Source: CAD feature listing. Evaluate the final solid. Frame: model axes, mm. A direction names the side the tool comes from. Round coordinates to 2 decimals unless told otherwise and drop trailing zeros. Order: outer loops, then holes, each group sorted by start corner. A loop starts at its lowest first (then second) coordinate and runs counter-clockwise, first axis right, second up. Notation, with made-up numbers: (12, 77) - (65, 77) arc R13 cw to (65, 88) - close; hole circle Ø4 at (26.25, 61). An arc over 180 degrees is marked (long way). Put each result on its own line as item: value. Start each with the question number.
1) Contact query for flat-ended pins moving along their axis: P1, Ø1.4, axis at x = 42, y = -207.5, coming from the +Z side; P2, Ø4, axis at y = -32.5, z = 39, coming from the -X side (3 decimals); P3, Ø8.5, axis at x = 48.5, z = 36.5, coming from the +Y side. Output: stop coordinate, or through.
2) Section B-B on z = 12. State how many separate pieces and enclosed holes the cut face has, then the cut area to 3 significant figures.
3) Access query for faces 1 (the face through (19, -96, 24.384)), 2 (the face through (31.75, -63, 4)), 3 (the face through (43.18, -90, 14)). Directions: +Z, -Z, +X, -X, +Y, -Y. A direction counts if a zero-diameter tool reaches every point of the face in a straight line with its end or side. Return the directions, or none.
4) Mould query, pull axis Y, two halves, no side actions, for faces 4 (the face through (20, -55.88, 17)), 5 (the face through (43.18, -203, 39)), 6 (the face through (32.258, -160, 12)), 7 (the face through (47, -177.8, 37)). Classes: +Y half, -Y half, draft (parallel to the pull), parting line (faces both ways), or undercut.
5) Line query: probe 1 along Y at (x, z) = (11, 14.5); probe 2 along X at (y, z) = (-203, 19); probe 3 along X at (y, z) = (-187, 5.5). Output: solid intervals per line, ascending. Write a range as [from, to].
6) Section C-C on z = 41. Output: boundary loops of the cut face in (x, y) (3 decimals).
7) Section D-D on x = 16. Output: boundary loops of the cut face in (y, z), then the cut area to 3 significant figures.
8) Section A-A on y = -203.2. Output: boundary loops of the cut face in (x, z).
```python
from build123d import *

# Parameters (mm, degrees)
F0_W            = 50.8
F0_H            = 44.45
F3_DEPTH        = 228.6
F4_SIZE2        = 12.7
F4_SIZE         = 25.4
F1_W            = 27.178
F1_H            = 8.89
F5_DEPTH        = 228.6
F2_W            = 4.572
F2_H            = 10.16
F6_DEPTH        = 228.6
F8_DEPTH        = 24.384
F9_W            = 2.364222
F9_H            = 0.78807
F10_DEPTH       = 12.192
F12_DEPTH       = 35.56
F14_D           = 6.35
F14_CBORE_D     = 16.51
F14_CBORE_DEPTH = 35.56


with BuildPart() as f3:
    # F0 (on Front) → F3 (new body)
    with BuildSketch(Plane.XZ):
        with Locations((25.4, 22.225)):
            Rectangle(F0_W, F0_H)
    extrude(amount=F3_DEPTH)

    # F4
    f4_edges = [f3.edges().sort_by_distance(p)[0] for p in [
        (0, -114.3, 44.45),
    ]]
    chamfer(f4_edges, length=F4_SIZE, length2=F4_SIZE2)

    # F1 (on Front) → F5 (cut)
    with BuildSketch(Plane.XZ):
        with Locations((18.161, 4.445)):
            Rectangle(F1_W, F1_H)
    extrude(amount=F5_DEPTH, mode=Mode.SUBTRACT)

    # F2 (on Front) → F6 (cut)
    with BuildSketch(Plane.XZ):
        with Locations((40.894, 39.37)):
            Rectangle(F2_W, F2_H)
    extrude(amount=F6_DEPTH, mode=Mode.SUBTRACT)

    # F7 (on face) → F8 (cut)
    with BuildSketch(Plane(origin=(0, 0, 0), x_dir=(1, 0, 0), z_dir=(0, 0, -1))):
        with BuildLine():
            ThreePointArc((32.258, 53.34), (31.514051, 55.136051), (29.718, 55.88))
            Line((29.718, 55.88), (9.398, 55.88))
            ThreePointArc((9.398, 55.88), (7.601949, 55.136051), (6.858, 53.34))
            Line((6.858, 53.34), (6.858, 7.62))
            ThreePointArc((6.858, 7.62), (7.601949, 5.823949), (9.398, 5.08))
            Line((9.398, 5.08), (29.718, 5.08))
            ThreePointArc((29.718, 5.08), (31.514051, 5.823949), (32.258, 7.62))
            Line((32.258, 7.62), (32.258, 53.34))
        make_face()
        with BuildLine():
            ThreePointArc((32.258, 118.11), (31.514051, 119.906051), (29.718, 120.65))
            Line((29.718, 120.65), (9.398, 120.65))
            ThreePointArc((9.398, 120.65), (7.601949, 119.906051), (6.858, 118.11))
            Line((6.858, 118.11), (6.858, 72.39))
            ThreePointArc((6.858, 72.39), (7.601949, 70.593949), (9.398, 69.85))
            Line((9.398, 69.85), (29.718, 69.85))
            ThreePointArc((29.718, 69.85), (31.514051, 70.593949), (32.258, 72.39))
            Line((32.258, 72.39), (32.258, 118.11))
        make_face()
        with BuildLine():
            ThreePointArc((32.258, 182.88), (31.514051, 184.676051), (29.718, 185.42))
            Line((29.718, 185.42), (9.398, 185.42))
            ThreePointArc((9.398, 185.42), (7.601949, 184.676051), (6.858, 182.88))
            Line((6.858, 182.88), (6.858, 137.16))
            ThreePointArc((6.858, 137.16), (7.601949, 135.363949), (9.398, 134.62))
            Line((9.398, 134.62), (29.718, 134.62))
            ThreePointArc((29.718, 134.62), (31.514051, 135.363949), (32.258, 137.16))
            Line((32.258, 137.16), (32.258, 182.88))
        make_face()
    extrude(amount=-F8_DEPTH, mode=Mode.SUBTRACT)

    # F9 (on face) → F10 (cut)
    with BuildSketch(Plane.YZ.offset(50.8)):
        with BuildLine():
            Line((0, 22.098), (0, 44.45))
            Line((0, 44.45), (-177.8, 44.45))
            Line((-177.8, 44.45), (-177.8, 28.448))
            ThreePointArc((-177.8, 28.448), (-175.940128, 23.957872), (-171.45, 22.098))
            Line((-171.45, 22.098), (0, 22.098))
        make_face()
        with Locations((10.441655, 33.889506)):
            Rectangle(F9_W, F9_H)
    extrude(amount=-F10_DEPTH, mode=Mode.SUBTRACT)

    # F11 (on face) → F12 (cut)
    with BuildSketch(Plane.XY.offset(44.45)):
        with BuildLine():
            Line((43.18, 0), (38.608, 0))
            Line((38.608, 0), (38.608, -177.8))
            ThreePointArc((38.608, -177.8), (39.277554, -179.416446), (40.894, -180.086))
            ThreePointArc((40.894, -180.086), (42.510446, -179.416446), (43.18, -177.8))
            Line((43.18, -177.8), (43.18, 0))
        make_face()
    extrude(amount=-F12_DEPTH, mode=Mode.SUBTRACT)

    # F14 (through all)
    with Locations(Plane(origin=(0, 0, 0), x_dir=(1, 0, 0), z_dir=(0, 0, -1))):
        with Locations((28.575, 203.2)):
            CounterBoreHole(F14_D / 2, F14_CBORE_D / 2, F14_CBORE_DEPTH)


solid = f3.part
```
Answer sheet:
1. P1: z = 34.29
1. P2: x = 8.975
1. P3: y = -177.8
2. separate pieces: 1
2. enclosed holes: 4
2. area: 6,720 mm^2
3. face 1: -Z
3. face 2: -Z, +Y, -Y
3. face 3: +Z, +Y
4. face 4: undercut
4. face 5: draft
4. face 6: undercut
4. face 7: +Y half
5. probe 1: [-228.6, -185.42], [-134.62, -120.65], [-69.85, -55.88], [-5.08, 0]
5. probe 2: [0, 20.32], [36.83, 50.8]
5. probe 3: [0, 4.57], [31.75, 50.8]
6. outline: (10.975, -228.6) - (38.608, -228.6) - (38.608, 0) - (10.975, 0) - close; (43.18, -228.6) - (50.8, -228.6) - (50.8, -177.8) - (43.18, -177.8) - close; hole circle Ø6.35 at (28.575, -203.2)
7. outline: (-228.6, 8.89) - (-185.42, 8.89) - (-185.42, 24.38) - (-134.62, 24.38) - (-134.62, 8.89) - (-120.65, 8.89) - (-120.65, 24.38) - (-69.85, 24.38) - (-69.85, 8.89) - (-55.88, 8.89) - (-55.88, 24.38) - (-5.08, 24.38) - (-5.08, 8.89) - (0, 8.89) - (0, 44.45) - (-228.6, 44.45) - close
7. area: 5,770 mm^2
8. outline: (0, 0) - (4.57, 0) - (4.57, 8.89) - (20.32, 8.89) - (20.32, 35.56) - (25.4, 35.56) - (25.4, 44.45) - (12.7, 44.45) - (0, 19.05) - close; (31.75, 35.56) - (36.83, 35.56) - (36.83, 0) - (50.8, 0) - (50.8, 44.45) - (43.18, 44.45) - (43.18, 34.29) - (38.61, 34.29) - (38.61, 44.45) - (31.75, 44.45) - close
